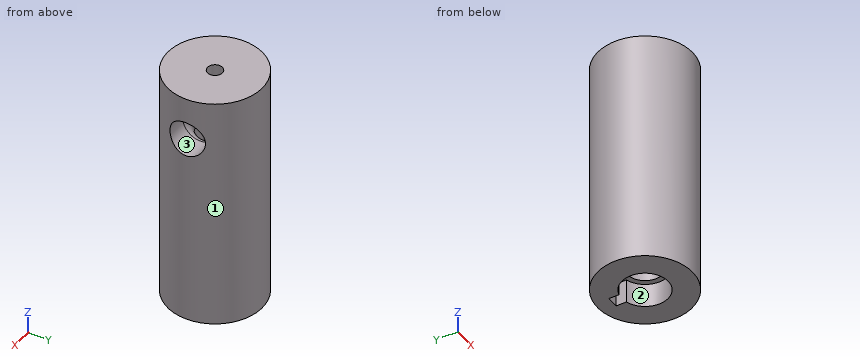
```python
from build123d import *

# Parameters (mm, degrees)
SKETCH1_R           = 20
BOSS_EXTRUDE1_DEPTH = 100
SKETCH3_R           = 3.15
CUT_EXTRUDE2_DEPTH  = 5
SKETCH2_R           = 7.5
SKETCH6_R           = 9.75
SKETCH6_W           = 5
SKETCH6_H           = 7.292344614
CUT_EXTRUDE3_DEPTH  = 10


with BuildPart() as part:
    # Sketch1 → Boss-Extrude1 (new body)
    with BuildSketch(Plane.XY):
        Circle(SKETCH1_R)
    extrude(amount=BOSS_EXTRUDE1_DEPTH)

    # Sketch3 → Cut-Extrude2 (cut)
    with BuildSketch(Plane.XY.offset(100)):
        Circle(SKETCH3_R)
    extrude(amount=-CUT_EXTRUDE2_DEPTH, mode=Mode.SUBTRACT)

    # Cut-Sweep1: sweep along a path in Sketch4
    with BuildLine(Plane(origin=(0, 0, 0), x_dir=(1, 0, 0), z_dir=(0, 1, 0))) as cut_sweep1_path:
        Line((0, 0), (0, -71.793883449))
        ThreePointArc((0, -71.793883449), (2.928932188, -78.864951261), (10, -81.793883449))
        Line((10, -81.793883449), (20, -81.793883449))
    # Sketch2 → Cut-Sweep1 (sweep, cut)
    with BuildSketch(Plane(origin=(0, 0, 0), x_dir=(-1, 0, 0), z_dir=(0, 0, -1))):
        Circle(SKETCH2_R)
    sweep(path=cut_sweep1_path.line, mode=Mode.SUBTRACT)

    # Sketch6 → Cut-Extrude3 (cut)
    with BuildSketch(Plane.XY):
        Circle(SKETCH6_R)
        with Locations((0, 10.103827693)):
            Rectangle(SKETCH6_W, SKETCH6_H)
    extrude(amount=CUT_EXTRUDE3_DEPTH, mode=Mode.SUBTRACT)


solid = part.part
```
Check sheet for the modelled part. Datum: model origin and axes. Units: mm. Face numbers are marked on the shaded views. Round coordinates to 2 decimals unless told otherwise and drop trailing zeros. Loops run counter-clockwise (first coordinate to the right, second up) from the corner with the lowest first, then second, coordinate; pieces in that order, holes last. Notation, with made-up numbers: (1, -38) -> (43, -38) arc R7 cw to (43, -28) -> close; hole circle Ø9 at (87, 36). An arc over 180 degrees is marked (long way). Write item = value, one per line. Start each with the question number.
1) Sectioned sample at A-A, the plane y = 0. Record the cut outline in (x, z), plus the area to 3 significant figures.
2) Sectioned sample at D-D, the plane y = 6.5. Record the cut outline in (x, z).
3) Thickness scan on probe 1 along Y at (x, z) = (0, 97); probe 2 along Z at (x, y) = (-6.5, -4.5); probe 3 along X at (y, z) = (-4.5, 73). Record the ranges inside material, lowest first.
4) Gauge pin test, flat ends, axial feed: pin 1 Ø3.5 at (y, z) = (11, 7.5) entering from +X; pin 2 Ø1 at (x, z) = (-7, 22.5) entering from -Y; pin 3 Ø5.5 at (x, z) = (-1, 3) entering from -Y. Record the tip position at first contact, or that the pin passes through.
5) Sectioned sample at C-C, the plane x = -16. Record the cut outline in (y, z), plus the area to 3 significant figures.
6) Release check for a two-part mould opening along X. For the marked faces 1, 2 and 3 record: released by +X, released by -X, zero draft, split by the parting line, or undercut.
7) Sectioned sample at B-B, the plane z = 7. Record the cut outline in (x, y).
Results are:
q1.outline = (-20, 0) -> (-9.75, 0) -> (-9.75, 10) -> (-7.5, 10) -> (-7.5, 71.79) arc R17.5 cw to (10, 89.29) -> (20, 89.29) -> (20, 100) -> (3.15, 100) -> (3.15, 95) -> (-3.15, 95) -> (-3.15, 100) -> (-20, 100) -> close; (7.5, 10) -> (9.75, 10) -> (9.75, 0) -> (20, 0) -> (20, 74.29) -> (10, 74.29) arc R2.5 ccw to (7.5, 71.79) -> close
q1.area = 2,460 mm^2
q2.outline = (-18.91, 0) -> (-7.27, 0) -> (-7.27, 10) -> (-3.74, 10) -> (-3.74, 71.79) arc R13.74 cw to (10, 85.54) -> (18.91, 85.54) -> (18.91, 100) -> (-18.91, 100) -> close; (3.74, 10) -> (7.27, 10) -> (7.27, 0) -> (18.91, 0) -> (18.91, 78.05) -> (10, 78.05) arc R6.26 ccw to (3.74, 71.79) -> close
q3.probe_1 = -20 to -3.15, 3.15 to 20
q3.probe_2 = 10 to 100
q3.probe_3 = -19.49 to -5.95, 6.19 to 19.49
q4.pin_1 = 17.73
q4.pin_2 = -18.91
q4.pin_3 = -20
q5.outline = (-12, 0) -> (12, 0) -> (12, 100) -> (-12, 100) -> close
q5.area = 2,400 mm^2
q6.face_1 = split by the parting line
q6.face_2 = undercut
q6.face_3 = zero draft
q7.outline = circle Ø40 at (0, 0); hole (-2.5, 9.42) arc R9.75 ccw (long way) to (2.5, 9.42) -> (2.5, 13.75) -> (-2.5, 13.75) -> close
